Source: CAD feature listing. Evaluate the final solid. Frame: model axes, mm. A direction names the side the tool comes from. Round coordinates to 2 decimals unless told otherwise and drop trailing zeros. Loops run counter-clockwise (first coordinate to the right, second up) from the corner with the lowest first, then second, coordinate; pieces in that order, holes last. Notation, with made-up numbers: M 26,-26 L 65,-26 A19 ccw 65,7 Z; hole C 26,16.25 d6. An arc over 180 degrees is marked long. One line per item, written item: value.
from build123d import *

# Parameters (mm, degrees)
SKETCH1_W           = 200
SKETCH1_H           = 90
SKETCH1_R           = 25
SKETCH1_R_2         = 3.25
SKETCH1_R_3         = 9
BOSS_EXTRUDE1_DEPTH = 4
FILLET1_R           = 5
SKETCH2_R           = 11
CUT_EXTRUDE1_DEPTH  = 6
SKETCH3_R           = 5
SKETCH3_R_2         = 6
CUT_EXTRUDE2_DEPTH  = 5


with BuildPart() as part:
    # Sketch1 → Boss-Extrude1 (new body, symmetric)
    with BuildSketch(Plane.XY):
        Rectangle(SKETCH1_W, SKETCH1_H)
        with Locations((-55, 0)):
            Circle(SKETCH1_R, mode=Mode.SUBTRACT)
        with Locations((-55, 32.5)):
            Circle(SKETCH1_R_2, mode=Mode.SUBTRACT)
        with Locations((-55, -32.5)):
            Circle(SKETCH1_R_2, mode=Mode.SUBTRACT)
        with Locations((-87.5, 0)):
            Circle(SKETCH1_R_2, mode=Mode.SUBTRACT)
        with Locations((-22.5, 0)):
            Circle(SKETCH1_R_2, mode=Mode.SUBTRACT)
        with Locations((55, 0)):
            Circle(SKETCH1_R_3, mode=Mode.SUBTRACT)
        with Locations((-90, 35)):
            Circle(SKETCH1_R_2, mode=Mode.SUBTRACT)
        with Locations((-20, 35)):
            Circle(SKETCH1_R_2, mode=Mode.SUBTRACT)
        with Locations((-90, -35)):
            Circle(SKETCH1_R_2, mode=Mode.SUBTRACT)
        with Locations((-20, -35)):
            Circle(SKETCH1_R_2, mode=Mode.SUBTRACT)
        with Locations((90, -35)):
            Circle(SKETCH1_R_2, mode=Mode.SUBTRACT)
        with Locations((20, -35)):
            Circle(SKETCH1_R_2, mode=Mode.SUBTRACT)
        with Locations((20, 35)):
            Circle(SKETCH1_R_2, mode=Mode.SUBTRACT)
        with Locations((90, 35)):
            Circle(SKETCH1_R_2, mode=Mode.SUBTRACT)
        with BuildLine():
            Line((3, 31), (3, 16))
            ThreePointArc((3, 16), (0, 13), (-3, 16))
            Line((-3, 16), (-3, 31))
            ThreePointArc((-3, 31), (0, 34), (3, 31))
        make_face(mode=Mode.SUBTRACT)
    extrude(amount=BOSS_EXTRUDE1_DEPTH, both=True)

    # Fillet1
    fillet1_edges = [part.edges().sort_by_distance(p)[0] for p in [
        (100, -45, 0),
        (-100, -45, 0),
        (-100, 45, 0),
        (100, 45, 0),
    ]]
    fillet(fillet1_edges, radius=FILLET1_R)

    # Sketch2 → Cut-Extrude1 (cut)
    with BuildSketch(Plane.XY.offset(4)):
        with Locations((55, 0)):
            Circle(SKETCH2_R)
    extrude(amount=-CUT_EXTRUDE1_DEPTH, mode=Mode.SUBTRACT)

    # Sketch3 → Cut-Extrude2 (cut)
    with BuildSketch(Plane.XY.offset(4)):
        with Locations((-90, 35)):
            Circle(SKETCH3_R)
        with Locations((-20, 35)):
            Circle(SKETCH3_R)
        with Locations((-90, -35)):
            Circle(SKETCH3_R)
        with Locations((-20, -35)):
            Circle(SKETCH3_R)
        with Locations((20, -35)):
            Circle(SKETCH3_R)
        with Locations((90, -35)):
            Circle(SKETCH3_R)
        with Locations((90, 35)):
            Circle(SKETCH3_R)
        with Locations((20, 35)):
            Circle(SKETCH3_R)
        with Locations((-55, 32.5)):
            Circle(SKETCH3_R_2)
        with Locations((-87.5, 0)):
            Circle(SKETCH3_R_2)
        with Locations((-55, -32.5)):
            Circle(SKETCH3_R_2)
        with Locations((-22.5, 0)):
            Circle(SKETCH3_R_2)
    extrude(amount=-CUT_EXTRUDE2_DEPTH, mode=Mode.SUBTRACT)


solid = part.part
1. Pull-direction query (X, two-part tool) for faces 1 (the face through (-99, -43, 0)), 2 (the face through (-1, 45, 0)), 3 (the face through (-27.26, -3.65, 1.54)); classes: released by +X, released by -X, zero draft, split by the parting line, or undercut.
Report:
face 1: released by -X
face 2: zero draft
face 3: undercut
2. Pin query (flat end, axial travel): pin 1 (6 mm diameter, centred on x = -20, y = 35, fed in from +Z); pin 2 (3 mm diameter, centred on x = 92.5, y = -36.5, fed in from +Z). Return the tip coordinate at first contact, or that it passes through.
Report:
pin 1: passes through
pin 2: stops at z = -1
3. Reachability of faces 4 (the face through (-19, -38.3, -1)), 5 (the face through (19.295, 31.827, -2.521)) from +Z, -Z, +X, -X, +Y, -Y: full face, straight path, thin tool, end or side. Return the list, or none.
Report:
face 4: +Z
face 5: +Z, -Z
4. Ray query, line 1 (Y direction, x = 20, z = 2.2); line 2 (Y direction, x = -55, z = -2.3); line 3 (Y direction, x = 55, z = -2.35). Return the intervals inside material, ascending. Write a range as [from, to].
Report:
line 1: y = [-45, -40], [-30, 30], [40, 45]
line 2: y = [-45, -35.75], [-29.25, -25], [25, 29.25], [35.75, 45]
line 3: y = [-45, -9], [9, 45]
5. Section query A-A (x = 55). Return the cut outline in (y, z), and give its area (3 significant figures).
Report:
outline: M -45,-4 L -9,-4 L -9,-2 L -11,-2 L -11,4 L -45,4 Z; M 9,-4 L 45,-4 L 45,4 L 11,4 L 11,-2 L 9,-2 Z
area: 552 mm2
6. Section query D-D (y = -22). Return the cut outline in (x, z), and give its area (3 significant figures).
Report:
outline: M -100,-4 L -66.87,-4 L -66.87,4 L -100,4 Z; M -43.13,-4 L 100,-4 L 100,4 L -43.13,4 Z
area: 1,410 mm2
7. Section query B-B (y = 0). Count the separate pieces of the cut face and the enclosed holes in it, and give its area (3 significant figures).
Report:
separate pieces: 5
enclosed holes: 0
area: 873 mm2
8. Section query C-C (x = 90). Return the cut outline in (y, z), and give its area (3 significant figures).
Report:
outline: M -45,-4 L -38.25,-4 L -38.25,-1 L -40,-1 L -40,4 L -45,4 Z; M -31.75,-4 L 31.75,-4 L 31.75,-1 L 30,-1 L 30,4 L -30,4 L -30,-1 L -31.75,-1 Z; M 38.25,-4 L 45,-4 L 45,4 L 40,4 L 40,-1 L 38.25,-1 Z
area: 581 mm2
